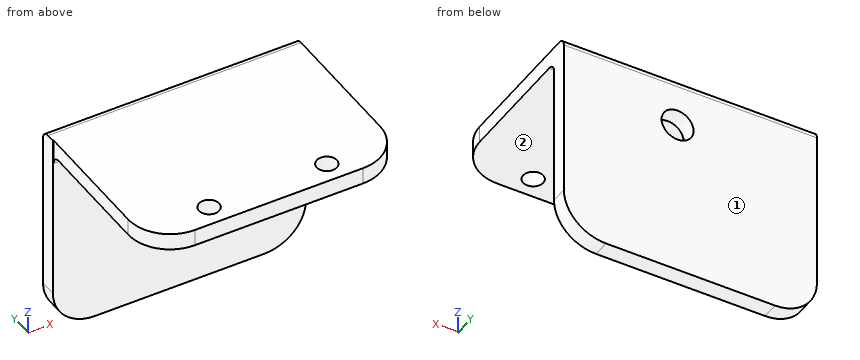
from build123d import *

# Parameters (mm, degrees)
SKETCH2_W           = 30
SKETCH2_H           = 22
BOSS_EXTRUDE1_DEPTH = 2
SKETCH3_W           = 30.097036207
SKETCH3_H           = 25
BOSS_EXTRUDE2_DEPTH = 2
SKETCH4_R           = 1.2
CUT_EXTRUDE1_DEPTH  = 2
FILLET1_R           = 1
FILLET2_R           = 1
FILLET3_R           = 5
FILLET4_R           = 5
SKETCH5_R           = 1.9
CUT_EXTRUDE2_DEPTH  = 2


with BuildPart() as part:
    # Sketch2 → Boss-Extrude1 (new body)
    with BuildSketch(Plane.XY):
        with Locations((-12.375323898, 10.6)):
            Rectangle(SKETCH2_W, SKETCH2_H)
    extrude(amount=BOSS_EXTRUDE1_DEPTH)

    # Sketch3 → Boss-Extrude2 (add)
    with BuildSketch(Plane(origin=(0, 21.6, 0), x_dir=(1, 0, 0), z_dir=(0, 1, 0))):
        with Locations((-12.423842002, 10.5)):
            Rectangle(SKETCH3_W, SKETCH3_H)
    extrude(amount=-BOSS_EXTRUDE2_DEPTH)

    # Sketch4 → Cut-Extrude1 (cut)
    with BuildSketch(Plane.XY.offset(2)):
        with Locations((-5.2, 2.1)):
            Circle(SKETCH4_R)
        with Locations((-19.2, 2.1)):
            Circle(SKETCH4_R)
    extrude(amount=-CUT_EXTRUDE1_DEPTH, mode=Mode.SUBTRACT)

    # Fillet1
    fillet1_edges = [part.edges().sort_by_distance(p)[0] for p in [
        (-12.375323898, 19.6, 0),
    ]]
    fillet(fillet1_edges, radius=FILLET1_R)

    # Fillet2
    fillet2_edges = [part.edges().sort_by_distance(p)[0] for p in [
        (-12.423842002, 21.6, 2),
    ]]
    fillet(fillet2_edges, radius=FILLET2_R)

    # Fillet3
    fillet3_edges = [part.edges().sort_by_distance(p)[0] for p in [
        (2.624676102, -0.4, 1),
        (-27.375323898, -0.4, 1),
    ]]
    fillet(fillet3_edges, radius=FILLET3_R)

    # Fillet4
    fillet4_edges = [part.edges().sort_by_distance(p)[0] for p in [
        (2.624676102, 20.6, -23),
        (-27.472360105, 20.6, -23),
    ]]
    fillet(fillet4_edges, radius=FILLET4_R)

    # Sketch5 → Cut-Extrude2 (cut)
    with BuildSketch(Plane(origin=(0, 21.6, 0), x_dir=(1, 0, 0), z_dir=(0, 1, 0))):
        with Locations((-10.890638189, 4.027670227)):
            Circle(SKETCH5_R)
    extrude(amount=-CUT_EXTRUDE2_DEPTH, mode=Mode.SUBTRACT)


solid = part.part
Build history of the part. All positions in model axes, mm. Face numbers are marked on the shaded views. A direction names the side the tool comes from. Give positions to 0.01 mm unless a question says otherwise; leave off trailing zeros. Loops run counter-clockwise (first coordinate to the right, second up) from the corner with the lowest first, then second, coordinate; pieces in that order, holes last. Notation, with made-up numbers: (-9.5, 85) - (0.5, 85) arc R20 cw to (0.5, 93) - close; hole circle Ø2 at (-36, 4.25). An arc over 180 degrees is marked (long way). Write item = value, one per line. Start each with the question number.
1) Tool access for the marked faces 1 and 2: list every direction of +Z, -Z, +X, -X, +Y, -Y with a clear straight run to the whole face (end or side of a thin tool).
2) Band-saw the part on C-C on z = -3. Give the cut face in (x, y).
3) Probe probe 1 along Y at (x, z) = (-8, -6.25); probe 2 along Z at (x, y) = (-25, 2.5); probe 3 along X at (y, z) = (20.25, -5). List the from-to ranges inside material, lowest first. Write a range as from..to.
4) Band-saw the part on A-A on x = -19.2. Give the cut face in (y, z).
5) Drop flat-ended pins along their axis: pin 1 Ø4 at (x, y) = (-5, 12.5) entering from -Z; pin 2 Ø6 at (x, z) = (-10.89, -4.03) entering from -Y; pin 3 Ø0.9 at (y, z) = (15, 1) entering from -X. Give the stop position or say it passes through.
6) Band-saw the part on B-B on y = 2.1. Give the cut face in (x, z), plus the area to 3 significant figures.
7) Band-saw the part on D-D on y = 13.75. Give the cut face in (x, z).
Final values:
q1.face_1 = +Z, -Z, +X, -X, +Y
q1.face_2 = -Z, +X, -X, -Y
q2.outline = (-27.47, 19.6) - (-12.49, 19.6) - (-12.49, 21.6) - (-27.47, 21.6) - close; (-9.29, 19.6) - (2.62, 19.6) - (2.62, 21.6) - (-9.29, 21.6) - close
q3.probe_1 = 19.6..21.6
q3.probe_2 = 0..2
q3.probe_3 = -27.47..-12.52, -9.26..2.62
q4.outline = (-0.4, 0) - (0.9, 0) - (0.9, 2) - (-0.4, 2) - close; (3.3, 0) - (18.6, 0) arc R1 cw to (19.6, -1) - (19.6, -23) - (21.6, -23) - (21.6, 1) arc R1 ccw to (20.6, 2) - (3.3, 2) - close
q5.pin_1 = 0
q5.pin_2 = 19.6
q5.pin_3 = -27.38
q6.outline = (-26.71, 0) - (-20.4, 0) - (-20.4, 2) - (-26.71, 2) - close; (-18, 0) - (-6.4, 0) - (-6.4, 2) - (-18, 2) - close; (-4, 0) - (1.95, 0) - (1.95, 2) - (-4, 2) - close
q6.area = 47.7 mm²
q7.outline = (-27.38, 0) - (2.62, 0) - (2.62, 2) - (-27.38, 2) - close
